Print and shaded views of the part. All mm, measured from the part's lowest x, y and z. Round coordinates to 2 decimals unless told otherwise and drop trailing zeros. Write each loop counter-clockwise with the first axis right and the second up, starting at its lowest first coordinate (ties: lowest second). Pieces come first, ordered by that corner, then holes. Notation, with made-up numbers: (60.5, 85.25) - (72.5, 85.25) arc R18 ccw to (72.5, 110.25) - close; hole circle Ø7 at (4, -27). An arc over 180 degrees is marked (long way). Put each result on its own line as item: value. Start each with the question number.
Item 1: Cut at D-D (z = 87.5). Give the cut face in (x, y) (1 decimal).
Item 2: Cut at B-B (z = 50.8). Give the cut face in (x, y) (1 decimal).
Item 3: Drill centre lines: line 1 (Z direction, x = 19.05, y = 1.6); line 2 (X direction, y = 0.4, z = 19.5); line 3 (X direction, y = 0.9, z = 21.5). Where is each one in solid material? Low to high. Write a range as from..to.
Item 4: Pin check, flat tip, straight feed: pin 1 Ø2 at (x, z) = (93, 19.5) entering from -Y. Stop position of the tip, or through.
Item 5: Cut at C-C (y = 2.5). Count the separate pieces of the cut face and the enclosed holes in it, and give its area (3 significant figures).
Item 6: Cut at A-A (x = 19.05). Give the cut face in (y, z) (1 decimal), and give its area (3 significant figures).
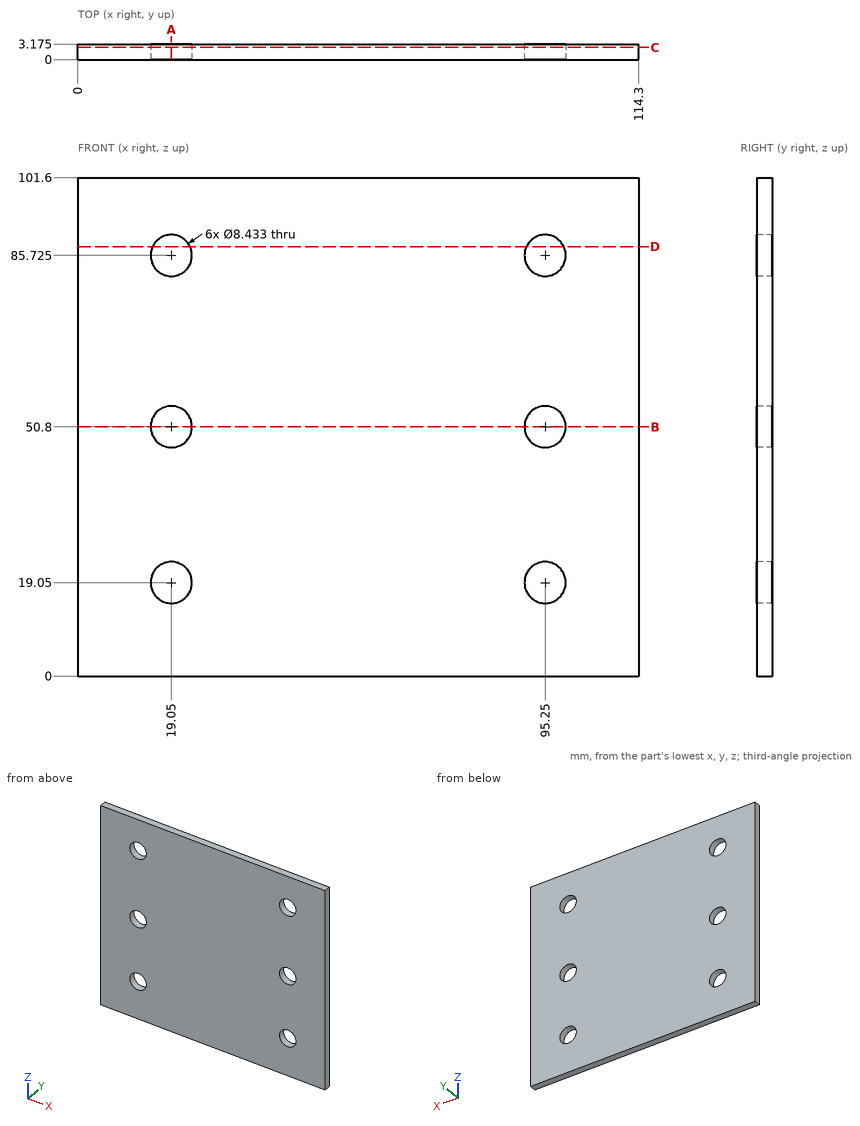
Output values:
1. outline: (0, 0) - (15.2, 0) - (15.2, 3.2) - (0, 3.2) - close; (22.9, 0) - (91.4, 0) - (91.4, 3.2) - (22.9, 3.2) - close; (99.1, 0) - (114.3, 0) - (114.3, 3.2) - (99.1, 3.2) - close
2. outline: (0, 0) - (14.8, 0) - (14.8, 3.2) - (0, 3.2) - close; (23.3, 0) - (91, 0) - (91, 3.2) - (23.3, 3.2) - close; (99.5, 0) - (114.3, 0) - (114.3, 3.2) - (99.5, 3.2) - close
3. line 1: 0..14.83, 23.27..46.58, 55.02..81.51, 89.94..101.6
3. line 2: 0..14.86, 23.24..91.06, 99.44..114.3
3. line 3: 0..15.62, 22.48..91.82, 98.68..114.3
4. pin 1: through
5. separate pieces: 1
5. enclosed holes: 6
5. area: 11,300 mm2
6. outline: (0, 0) - (3.2, 0) - (3.2, 14.8) - (0, 14.8) - close; (0, 23.3) - (3.2, 23.3) - (3.2, 46.6) - (0, 46.6) - close; (0, 55) - (3.2, 55) - (3.2, 81.5) - (0, 81.5) - close; (0, 89.9) - (3.2, 89.9) - (3.2, 101.6) - (0, 101.6) - close
6. area: 242 mm2
